Autodesk Inventor part; units mm, degrees
ref_plane "YZ Plane" through (0, 0, 0) normal (1, 0, 0) x (0, 1, 0)
ref_plane "XZ Plane" through (0, 0, 0) normal (0, 1, 0) x (-1, 0, 0)
ref_plane "XY Plane" through (0, 0, 0) normal (0, 0, 1) x (1, 0, 0)
sketch "Sketch1" plane through (0, 0, 0) normal (0, 1, 0) x (-1, 0, 0)
  line L0 (0, 0) -> (25.4, 0)
  line L1 (25.4, 0) -> (25.4, 25.4)
  line L2 (25.4, 25.4) -> (0, 25.4)
  line L3 (0, 25.4) -> (0, 0)
  line L4 (3.175, 22.225) -> (22.225, 22.225)
  line L5 (22.225, 22.225) -> (22.225, 3.175)
  line L6 (22.225, 3.175) -> (3.175, 3.175)
  line L7 (3.175, 3.175) -> (3.175, 22.225)
  dimension "d0" = 25.4
  dimension "d1" = 25.4
  dimension "d2" = 3.175
  dimension "d3" = 3.175
  dimension "d4" = 3.175
  dimension "d5" = 3.175
extrude "Extrusion1" add sketch "Sketch1" along normal blind 152.4
sketch "Sketch2" plane through (-25.4, 0, 25.4) normal (0, 0, 1) x (1, 0, 0)
  circle A0 centre (12.7, 139.7) radius 3.175
  line L0 (0, 152.4) -> (25.4, 152.4)
  line L1 (0, 0) -> (0, 152.4)
  point P0 (25.4, 0)
  dimension "d8" = 6.35
  dimension "d9" = 12.7
  dimension "d10" = 12.7
extrude "Extrusion2" cut sketch "Sketch2" against normal blind 152.4
sketch "Sketch3" plane through (-25.4, 0, 0) normal (-1, 0, 0) x (0, 0, 1)
  line L0 (0, 0) -> (0, 152.4)
  line L1 (0, 127) -> (0, 82.55) construction
  line L2 (-9.525, 127) -> (-9.525, 82.55)
  line L3 (9.525, 82.55) -> (9.525, 127)
  arc A0 (9.525, 127) -> (-9.525, 127) centre (0, 127) ccw
  arc A1 (-9.525, 82.55) -> (9.525, 82.55) centre (0, 82.55) ccw
  line L4 (0, 152.4) -> (25.4, 152.4)
  line L5 (0, 0) -> (25.4, 0)
  point P0 (0, 104.775)
  dimension "d13" = 44.45
  dimension "d14" = 19.05
  dimension "d15" = 25.4
  dimension "d16" = 82.55
extrude "Extrusion3" cut sketch "Sketch3" against normal blind 25.4
sketch "Sketch4" plane through (0, 0, 0) normal (0, 0, -1) x (-1, 0, 0)
  line L0 (0, 0) -> (25.4, 0)
  line L1 (25.4, 0) -> (25.4, 73.025)
  circle A0 centre (12.7, 38.1) radius 3.175
  circle A1 centre (12.7, 19.05) radius 3.175
  dimension "d19" = 19.05
  dimension "d20" = 12.7
  dimension "d21" = 12.7
  dimension "d22" = 19.05
  dimension "d23" = 6.35
  dimension "d24" = 6.35
extrude "Extrusion4" cut sketch "Sketch4" against normal blind 25.4
equation "\"d4\" = d2"
equation "\"d5\" = d3"
properties part number "6x1x1x0125 tube" material "Aluminum 6061"
Check sheet for the modelled part. Datum: model origin and axes. Units: mm. A direction names the side the tool comes from. Coordinates: 2 decimals unless noted, no trailing zeros. Loops run counter-clockwise (first coordinate to the right, second up) from the corner with the lowest first, then second, coordinate; pieces in that order, holes last. Notation, with made-up numbers: M 19.5,-36 L 55.5,-36 A18 ccw 55.5,-13 Z; hole C 89.5,-13 d7. An arc over 180 degrees is marked long. Answer as a JSON object with one key per item and string values.
1. Release check for a two-part mould opening along Z. For faces 4 (the cylindrical face through (-12.01, 15.95, 23.79)), 5 (the flat face through (-13, 75, 25.4)), 6 (the flat face through (-22.225, 75, 13)) record: pulls with the +Z half, pulls with the -Z half, needs draft (parallel to the pull), parting line crosses it, or undercut.
Outcome:
{"face 4": "needs draft", "face 5": "pulls with the +Z half", "face 6": "undercut"}
2. Sectioned sample at A-A on z = 18. Record the cut outline in (x, y) (3 decimals), and give its area (3 significant figures).
Outcome:
{"outline": "M -25.4,0 L -22.225,0 L -22.225,152.4 L -25.4,152.4 Z; M -3.175,0 L 0,0 L 0,152.4 L -3.175,152.4 Z", "area": "968 mm²"}
3. Depth check by flat-ended pin: P1, Ø1.5, axis at x = -21, z = 12.5, coming from the -Y side; P2, Ø1.6, axis at x = -24, y = 112.5, coming from the -Z side (3 decimals). Enter the tip coordinate at first touch or a pass-through.
Outcome:
{"P1": "through", "P2": "z = 9.525"}
4. Sectioned sample at B-B on y = 38.1. Record the cut outline in (x, z) (3 decimals).
Outcome:
{"outline": "M -25.4,0 L -15.875,0 L -15.875,3.175 L -22.225,3.175 L -22.225,22.225 L -15.875,22.225 L -15.875,25.4 L -25.4,25.4 Z; M -9.525,0 L 0,0 L 0,25.4 L -9.525,25.4 L -9.525,22.225 L -3.175,22.225 L -3.175,3.175 L -9.525,3.175 Z"}
5. Sectioned sample at D-D on y = 107. Record the cut outline in (x, z) (3 decimals), and give its area (3 significant figures).
Outcome:
{"outline": "M -25.4,9.525 L -22.225,9.525 L -22.225,22.225 L -3.175,22.225 L -3.175,9.525 L 0,9.525 L 0,25.4 L -25.4,25.4 Z", "area": "161 mm²"}
6. Access from +Z, -Z, +X, -X, +Y, -Y to the whole of each face (thin tool, end or side, straight path). Record for faces 1 (the flat face through (-25.4, 75, 13)), 2 (the flat face through (-2, 104, 9.525)), 3 (the flat face through (-9, 36, 3.175)).
Outcome:
{"face 1": "+Z, -Z, -X, +Y, -Y", "face 2": "-Z, +X, -X", "face 3": "+Y, -Y"}
7. Scan lines: L1, parallel to Y at x = -12.7, z = 23.35 (3 decimals); L2, parallel to Y at x = -14, z = 2.5; L3, parallel to Z at x = -16.75, y = 51 (3 decimals). Record each from-to range of solid material in increasing order. Write a range as from..to.
Outcome:
{"L1": "0..15.875, 22.225..34.925, 41.275..136.525, 142.875..152.4", "L2": "0..16.15, 21.95..35.2, 41..73.36, 136.19..136.8, 142.6..152.4", "L3": "0..3.175, 22.225..25.4"}
8. Sectioned sample at C-C on x = -6.25. Record the cut outline in (y, z) (3 decimals), and give its area (3 significant figures).
Outcome:
{"outline": "M 0,0 L 73.025,0 A9.525 cw 73.57,3.175 L 0,3.175 Z; M 0,22.225 L 152.4,22.225 L 152.4,25.4 L 0,25.4 Z; M 135.98,3.175 A9.525 cw 136.525,0 L 152.4,0 L 152.4,3.175 Z", "area": "767 mm²"}
